The model under review builds one solid part; all positions refer to its coordinate system, in mm. Face numbers are marked on the shaded views. A direction names the side the tool comes from. Coordinates: 2 decimals unless noted, no trailing zeros. Write each loop counter-clockwise with the first axis right and the second up, starting at its lowest first coordinate (ties: lowest second). Pieces come first, ordered by that corner, then holes. Notation, with made-up numbers: (-31.75, 33) - (-1.75, 33) arc R35 ccw to (-1.75, 70) - close; hole circle Ø2 at (3, -18.75). An arc over 180 degrees is marked (long way). Put each result on its own line as item: value.
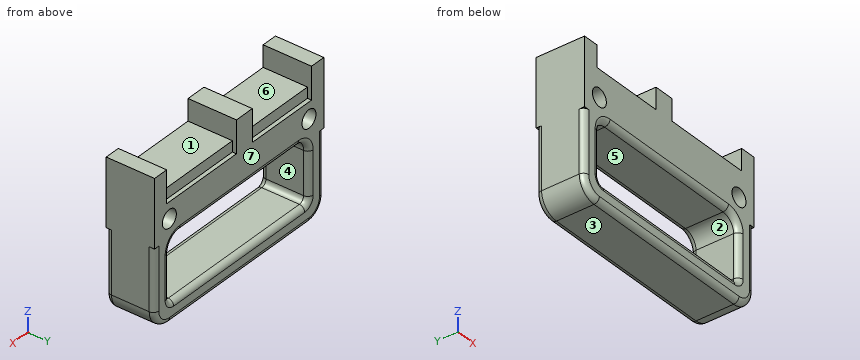
from build123d import *

# Parameters (mm, degrees)
F0_R     = 3.3
F1_DEPTH = 18
F2_W     = 33
F2_H     = 4
F2_W_2   = 28
F3_DEPTH = 1.5
F4_R     = 2
F5_W     = 5.8
F5_H     = 18
F5_W_2   = 5.7
F6_DEPTH = 25
F7_R     = 3.3
F8_DEPTH = 18.001


with BuildPart() as f1:
    # F0 (on Front) → F1 (new body)
    with BuildSketch(Plane.XZ):
        with BuildLine():
            Line((0, 25), (0, 0))
            Line((0, 0), (0, -23))
            ThreePointArc((0, -23), (2.050253, -27.949747), (7, -30))
            Line((7, -30), (73, -30))
            ThreePointArc((73, -30), (77.949747, -27.949747), (80, -23))
            Line((80, -23), (80, 0))
            Line((80, 0), (80, 25))
            Line((80, 25), (74.3, 25))
            Line((74.3, 25), (74.3, 17))
            Line((74.3, 17), (41.3, 17))
            Line((41.3, 17), (41.3, 25))
            Line((41.3, 25), (33.8, 25))
            Line((33.8, 25), (33.8, 17))
            Line((33.8, 17), (5.8, 17))
            Line((5.8, 17), (5.8, 25))
            Line((5.8, 25), (0, 25))
        make_face()
        with BuildLine():
            ThreePointArc((7, -5), (8.464466, -1.464466), (12, 0))
            Line((12, 0), (68, 0))
            ThreePointArc((68, 0), (71.535534, -1.464466), (73, -5))
            Line((73, -5), (73, -21))
            ThreePointArc((73, -21), (72.414214, -22.414214), (71, -23))
            Line((71, -23), (9, -23))
            ThreePointArc((9, -23), (7.585786, -22.414214), (7, -21))
            Line((7, -21), (7, -5))
        make_face(mode=Mode.SUBTRACT)
        with Locations((7, 7)):
            Circle(F0_R, mode=Mode.SUBTRACT)
        with Locations((73, 7)):
            Circle(F0_R, mode=Mode.SUBTRACT)
    extrude(amount=F1_DEPTH)

    # F2 (on face) → F3 (cut)
    with BuildSketch(Plane(origin=(0, 0, 0), x_dir=(-1, 0, 0), z_dir=(0, 1, 0))):
        with Locations((-57.8, 15)):
            Rectangle(F2_W, F2_H)
        with Locations((-19.8, 15)):
            Rectangle(F2_W_2, F2_H)
    extrude(amount=-F3_DEPTH, mode=Mode.SUBTRACT)

    # F4
    f4_edges = [f1.edges().sort_by_distance(p)[0] for p in [
        (72.414214, 0, -22.414214),
        (73, 0, -13),
        (7, -18, -13),
        (40, 0, -30),
        (0, -18, 1),
    ]]
    fillet(f4_edges, radius=F4_R)

    # F5 (on face) → F6 (join)
    with BuildSketch(Plane.XY.offset(25)):
        with Locations((2.9, -9)):
            Rectangle(F5_W, F5_H)
        with Locations((77.15, -9)):
            Rectangle(F5_W_2, F5_H)
    extrude(amount=-F6_DEPTH)

    # F7 (on face) → F8 (cut, through all)
    with BuildSketch(Plane.XZ.offset(18)):
        with Locations((73, 7)):
            Circle(F7_R)
        with Locations((7, 7)):
            Circle(F7_R)
    extrude(amount=-F8_DEPTH, mode=Mode.SUBTRACT)


solid = f1.part
1. Machinability: for the marked faces 1, 2 and 3, which of the approach directions +Z, -Z, +X, -X, +Y, -Y give a long, thin tool a straight path to every point of the face, cutting with its end or side? Answer none if there is none.
Determined:
face 1: +Z, +Y, -Y
face 2: +Y, -Y
face 3: -Z, +X, -X, +Y, -Y
2. Consider section D-D on z = -12. State the section outline as (x, y) points.
Determined:
outline: (0, -16) arc R2 ccw to (2, -18) - (5, -18) arc R2 ccw to (7, -16) - (7, -2) arc R2 ccw to (5, 0) - (2, 0) arc R2 ccw to (0, -2) - close; (73, -16) arc R2 ccw to (75, -18) - (78, -18) arc R2 ccw to (80, -16) - (80, -2) arc R2 ccw to (78, 0) - (75, 0) arc R2 ccw to (73, -2) - close
3. For pin 1 Ø1.6 at (x, y) = (15.5, -0.5) entering from +Z; pin 2 Ø0.6 at (x, y) = (78.5, -17) entering from -Z; pin 3 Ø5 at (x, y) = (43, -12.5) entering from +Z; pin 4 Ø6 at (x, z) = (73, 7) entering from +Y, all flat-tipped, find the tip position at first contact; note any pin that passes through.
Determined:
pin 1: stops at z = 13
pin 2: stops at z = -27.35
pin 3: stops at z = 25
pin 4: passes through
4. Consider section C-C on y = -12.5. State the section outline as (x, z) points.
Determined:
outline: (0, -23) arc R7 ccw to (7, -30) - (73, -30) arc R7 ccw to (80, -23) - (80, 25) - (74.3, 25) - (74.3, 17) - (41.3, 17) - (41.3, 25) - (33.8, 25) - (33.8, 17) - (5.8, 17) - (5.8, 25) - (0, 25) - close; hole circle Ø6.6 at (7, 7); hole (7, -21) arc R2 ccw to (9, -23) - (71, -23) arc R2 ccw to (73, -21) - (73, -5) arc R5 ccw to (68, 0) - (12, 0) arc R5 ccw to (7, -5) - close; hole circle Ø6.6 at (73, 7)
5. Consider section A-A on z = 7. State the section outline as (x, y) points, plus the area to 3 significant figures.
Determined:
outline: (0, -18) - (3.7, -18) - (3.7, 0) - (0, 0) - close; (10.3, -18) - (69.7, -18) - (69.7, 0) - (10.3, 0) - close; (76.3, -18) - (80, -18) - (80, 0) - (76.3, 0) - close
area: 1,200 mm^2
6. The part is to be moulded in two halves that separate along Z. For the marked faces 4, 5, 6 and 7, say which applies: +Z half, -Z half, draft (parallel to the pull), parting line (faces both ways), or undercut.
Determined:
face 4: undercut
face 5: undercut
face 6: +Z half
face 7: draft
7. Consider section B-B on x = 20. State the section outline as (y, z) points, plus the area to 3 significant figures.
Determined:
outline: (-18, -28) arc R2 ccw to (-16, -30) - (-2, -30) arc R2 ccw to (0, -28) - (0, -25) arc R2 ccw to (-2, -23) - (-16, -23) arc R2 ccw to (-18, -25) - close; (-18, 2) arc R2 ccw to (-16, 0) - (-2, 0) arc R2 ccw to (0, 2) - (0, 13) - (-1.5, 13) - (-1.5, 17) - (-18, 17) - close
area: 421 mm^2
8. To check wall thickness, follow probe 1 along X at (y, z) = (-6, 19); probe 2 along Z at (x, y) = (22, -15.5); probe 3 along Z at (x, y) = (9, -0.75). State the ranges of each line that lie inside material, in increasing order.
Determined:
probe 1: x = 0 to 5.8, 33.8 to 41.3, 74.3 to 80
probe 2: z = -30 to -23, 0 to 17
probe 3: z = -29.56 to -23.44, -0.46 to 4.38, 9.62 to 13
